Verification items for this drawing (mm, ordinates from the low corner). A direction names the side the tool comes from. Round coordinates to 2 decimals unless told otherwise and drop trailing zeros. Order: outer loops, then holes, each group sorted by start corner. A loop starts at its lowest first (then second) coordinate and runs counter-clockwise, first axis right, second up. Notation, with made-up numbers: M 19.25,68 L 51.25,68 A20 ccw 51.25,93 Z; hole C -3,81 d4. An arc over 180 degrees is marked long. One line per item, written item: value. Start each with the question number.
(1) Access from +Z, -Z, +X, -X, +Y, -Y to the whole of each face (thin tool, end or side, straight path). Record for the marked faces 1 and 2.
(2) Thickness scan on L1, parallel to Z at x = 111.5, y = 78; L2, parallel to Z at x = 83, y = 44; L3, parallel to Y at x = 68.5, z = 39 (1 decimal). Record the ranges inside material, lowest first.
(3) Cross-section at B-B, the plane y = 78.5. Enter the section's corners in (x, z), and give its area (3 significant figures).
(4) Depth check by flat-ended pin: pin 1 Ø3 at (x, z) = (71.5, 46.5) entering from -Y. Enter the tip coordinate at first touch or a pass-through.
(5) Cross-section at C-C, the plane z = 38.5. Enter the section's corners in (x, y), and give its area (3 significant figures).
(6) Cross-section at A-A, the plane x = 118. Enter the section's corners in (y, z), and give its area (3 significant figures).
(7) Cross-section at D-D, the plane x = 58. Enter the section's corners in (y, z) (1 decimal), and give its area (3 significant figures).
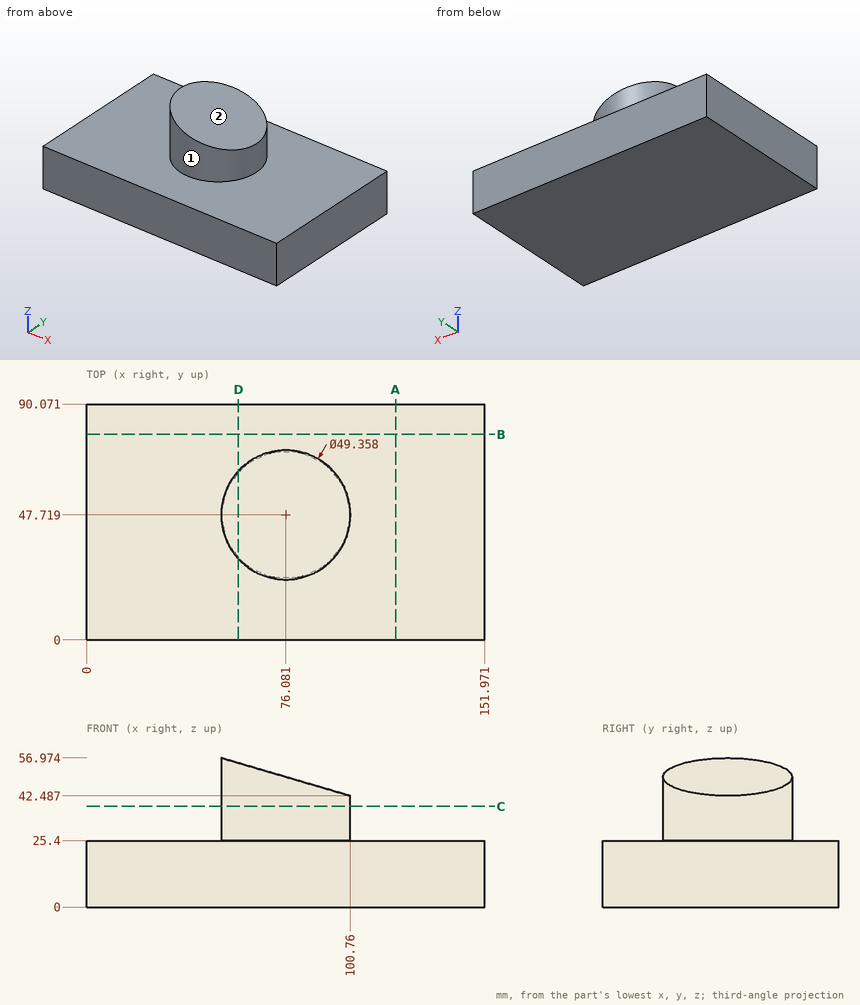
Values found:
1. face 1: +Z
1. face 2: +Z, +X, +Y, -Y
2. L1: 0 to 25.4
2. L2: 0 to 47.7
2. L3: 24.2 to 71.2
3. outline: M 0,0 L 151.97,0 L 151.97,25.4 L 0,25.4 Z
3. area: 3,860 mm^2
4. pin 1: y = 23.23
5. outline: C 76.08,47.72 d49.36
5. area: 1,910 mm^2
6. outline: M 0,0 L 90.07,0 L 90.07,25.4 L 0,25.4 Z
6. area: 2,290 mm^2
7. outline: M 0,0 L 90.1,0 L 90.1,25.4 L 64.5,25.4 L 64.5,55 L 30.9,55 L 30.9,25.4 L 0,25.4 Z
7. area: 3,280 mm^2
